from build123d import *

# Parameters (mm, degrees)
SKETCH1_R                     = 55
BOSS_EXTRUDE2_DEPTH           = 20
SKETCH2_R                     = 51
CUT_EXTRUDE1_DEPTH            = 17
SKETCH10_R                    = 1.5
BOSS_EXTRUDE3_DEPTH           = 10
SKETCH10_3_W                  = 7
SKETCH10_3_H                  = 7
CUT_EXTRUDE4_DEPTH            = 10
FILLET1_R                     = 3
SKETCH11_R                    = 4
BOSS_EXTRUDE4_DEPTH           = 20
TAP_DRILL_FOR_4_40_TAP1_D     = 2.2606
TAP_DRILL_FOR_4_40_TAP1_DEPTH = 13.05
TAP_DRILL_FOR_4_40_TAP1_TIP   = 0.679152758
SKETCH14_R                    = 2.5
CUT_EXTRUDE5_DEPTH            = 50


with BuildPart() as part:
    # Sketch1 → Boss-Extrude2 (new body)
    with BuildSketch(Plane.XY):
        with Locations((328.389379834, 629.271631436)):
            Circle(SKETCH1_R)
    extrude(amount=BOSS_EXTRUDE2_DEPTH)

    # Sketch2 → Cut-Extrude1 (cut)
    with BuildSketch(Plane(origin=(0, 0, 0), x_dir=(-1, 0, 0), z_dir=(0, 0, -1))):
        with Locations((-328.628637891, 629.384320649)):
            Circle(SKETCH2_R)
    extrude(amount=-CUT_EXTRUDE1_DEPTH, mode=Mode.SUBTRACT)

    # Sketch10 → Boss-Extrude3 (add)
    with BuildSketch(Plane(origin=(0, 0, 17), x_dir=(-1, 0, 0), z_dir=(0, 0, -1))):
        with Locations((-374.389379834, 627.076422512)):
            Circle(SKETCH10_R)
        with Locations((-282.389379834, 627.076422512)):
            Circle(SKETCH10_R)
    extrude(amount=BOSS_EXTRUDE3_DEPTH)

    # Sketch10<3> → Cut-Extrude4 (cut)
    with BuildSketch(Plane(origin=(0, 0, 17), x_dir=(-1, 0, 0), z_dir=(0, 0, -1))):
        with Locations((-328.389379834, 627.076422512)):
            Rectangle(SKETCH10_3_W, SKETCH10_3_H)
        with Locations((-310.889379834, 627.076422512)):
            Rectangle(SKETCH10_3_W, SKETCH10_3_H)
        with Locations((-293.389379834, 627.076422512)):
            Rectangle(SKETCH10_3_W, SKETCH10_3_H)
        with Locations((-345.889379834, 627.076422512)):
            Rectangle(SKETCH10_3_W, SKETCH10_3_H)
        with Locations((-363.389379834, 627.076422512)):
            Rectangle(SKETCH10_3_W, SKETCH10_3_H)
    extrude(amount=-CUT_EXTRUDE4_DEPTH, mode=Mode.SUBTRACT)

    # Fillet1
    fillet1_edges = [part.edges().sort_by_distance(p)[0] for p in [
        (273.389379834, 629.271631436, 20),
    ]]
    fillet(fillet1_edges, radius=FILLET1_R)

    # Sketch11 → Boss-Extrude4 (add)
    with BuildSketch(Plane(origin=(0, 0, 17), x_dir=(-1, 0, 0), z_dir=(0, 0, -1))):
        with Locations((-306.628637891, 665.384320649)):
            Circle(SKETCH11_R)
        with Locations((-350.628637891, 665.384320649)):
            Circle(SKETCH11_R)
        with Locations((-350.628637891, 593.384320649)):
            Circle(SKETCH11_R)
        with Locations((-306.628637891, 593.384320649)):
            Circle(SKETCH11_R)
    extrude(amount=BOSS_EXTRUDE4_DEPTH)

    # Tap Drill for #4-40 Tap1
    with Locations(Plane(origin=(0, 0, -3), x_dir=(-1, 0, 0), z_dir=(0, 0, -1))):
        with Locations((-350.628637891, 665.384320649), (-306.628637891, 665.384320649), (-350.628637891, 593.384320649), (-306.628637891, 593.384320649)):
            Hole(TAP_DRILL_FOR_4_40_TAP1_D / 2, depth=TAP_DRILL_FOR_4_40_TAP1_DEPTH)
            with Locations((0, 0, -(TAP_DRILL_FOR_4_40_TAP1_DEPTH + TAP_DRILL_FOR_4_40_TAP1_TIP / 2))):  # 118° drill point
                Cone(0, TAP_DRILL_FOR_4_40_TAP1_D / 2, TAP_DRILL_FOR_4_40_TAP1_TIP, mode=Mode.SUBTRACT)

    # Sketch14 → Cut-Extrude5 (cut)
    with BuildSketch(Plane(origin=(0, 623.576422512, 0), x_dir=(1, 0, 0), z_dir=(0, 1, 0))):
        with Locations((330.379647502, 0)):
            Circle(SKETCH14_R)
    extrude(amount=-CUT_EXTRUDE5_DEPTH, mode=Mode.SUBTRACT)


solid = part.part
Design review of the part built by this model. Coordinates are the model's own, in mm. A direction names the side the tool comes from. Round coordinates to 2 decimals unless told otherwise and drop trailing zeros. One line per item, written item: value. Start each with the question number.
1. Clearance check with flat-ended pins moving along their axes: P1, Ø3, axis at y = 669.5, z = 11, coming from the -X side; P2, Ø2.5, axis at y = 625.5, z = 18, coming from the -X side; P3, Ø1, axis at x = 367.5, y = 642, coming from the -Z side; P4, Ø2.5, axis at x = 350.63, y = 593.38, coming from the -Z side. State where each tip first meets the part, or that it passes through.
2. Draft analysis for pull direction Y (two halves, no side actions). For faces 1 (the face through (324.889, 627, 18)), 2 (the face through (316.47, 575.58, 8.38)), 3 (the face through (303.7, 584.7, 0)), state which applies: pulls with the +Y half, pulls with the -Y half, needs draft (parallel to the pull), parting line crosses it, or undercut.
3. To check wall thickness, follow probe 1 along X at (y, z) = (663, 7.5); probe 2 along Y at (x, z) = (305, 8.5); probe 3 along X at (y, z) = (665, -1.75). State the ranges of each line that lie inside material, in increasing order. Write a range as from..to.
4. For faces 4 (the face through (328, 623.576, 18)), 5 (the face through (330.3, 576.4, 2.5)), 6 (the face through (346.934, 591.852, 7.14)), list the 3-axis set-ups (+Z, -Z, +X, -X, +Y, -Y) from which the entire face can be reached by the end or side of a thin tool; tool diameter is ignored.
5. Take a section at A-A on z = 8.75. State how many separate pieces and enclosed holes the cut face has, then the cut area to 3 significant figures.
Computed:
1. P1: stops at x = 289.34
1. P2: stops at x = 273.47
1. P3: stops at z = 17
1. P4: stops at z = -3
2. face 1: undercut
2. face 2: parting line crosses it
2. face 3: needs draft
3. probe 1: x = 284.95..290.28, 303.42..309.84, 347.42..353.84, 366.98..371.83
3. probe 2: y = 579.49..584.19, 589.73..597.04, 661.73..669.04, 674.58..679.05
3. probe 3: x = 302.65..305.57, 307.69..310.61, 346.65..349.57, 351.69..354.61
4. face 4: +Z, -Z
4. face 5: -Z, -Y
4. face 6: -Z
5. separate pieces: 7
5. enclosed holes: 5
5. area: 1,530 mm²
